from build123d import *

# Parameters (mm, degrees)
EXTRUDE_1_DEPTH   = 20
EXTRUDE_1_2_DEPTH = 55


with BuildPart() as part:
    # 草图1 → Extrude 1 (new body)
    with BuildSketch(Plane(origin=(0, 0, 0), x_dir=(1, 0, 0), z_dir=(0, 1, 0))):
        with BuildLine():
            Line((-50.205761317, 12.5), (49.794238683, 12.5))
            ThreePointArc((49.794238683, 12.5), (62.294238683, 0), (49.794238683, -12.5))
            Line((49.794238683, -12.5), (-50.205761317, -12.5))
            ThreePointArc((-50.205761317, -12.5), (-62.705761317, 0), (-50.205761317, 12.5))
        make_face()
    extrude(amount=EXTRUDE_1_DEPTH)

    # 草图2 → Extrude 1 2 (add)
    with BuildSketch(Plane(origin=(0, 20, 0), x_dir=(1, 0, 0), z_dir=(0, 1, 0))):
        with BuildLine():
            Line((49.794238683, 12.5), (-50.205761317, 12.5))
            ThreePointArc((-50.205761317, 12.5), (-62.705761317, 0), (-50.205761317, -12.5))
            Line((-50.205761317, -12.5), (49.794238683, -12.5))
            ThreePointArc((49.794238683, -12.5), (62.294238683, 0), (49.794238683, 12.5))
        make_face()
        with BuildLine():
            Line((49.794238683, 7.5), (-50.205761317, 7.5))
            ThreePointArc((-50.205761317, 7.5), (-57.705761317, 0), (-50.205761317, -7.5))
            Line((-50.205761317, -7.5), (49.794238683, -7.5))
            ThreePointArc((49.794238683, -7.5), (57.294238683, 0), (49.794238683, 7.5))
        make_face(mode=Mode.SUBTRACT)
    extrude(amount=EXTRUDE_1_2_DEPTH)


solid = part.part
Source: CAD feature listing. Evaluate the final solid. Frame: model axes, mm. A direction names the side the tool comes from. Round coordinates to 2 decimals unless told otherwise and drop trailing zeros. Order: outer loops, then holes, each group sorted by start corner. A loop starts at its lowest first (then second) coordinate and runs counter-clockwise, first axis right, second up. Notation, with made-up numbers: (38.25, -16) - (46.25, -16) arc R20 cw to (46.25, 23) - close; hole circle Ø9 at (-29, 1.5). An arc over 180 degrees is marked (long way). Use a Markdown table: item, result. Add a question column.
1. Line query: probe 1 along Z at (x, y) = (-15, 55.5); probe 2 along X at (y, z) = (59.5, -2); probe 3 along Y at (x, z) = (-7, -1.5). Output: solid intervals per line, ascending.
2. Set-up query: faces 4 (the cylindrical face through (-62.703, 36.975, -0.275)), 5 (the cylindrical face through (57.292, 47.115, 0.165)). Return all of +Z, -Z, +X, -X, +Y, -Y with unobstructed straight access to the full face (end or side cutting, diameter ignored); none if empty.
3. Section query B-B (y = 49.5). Return the cut outline in (x, z).
4. Section query A-A (x = -38). Return the cut outline in (y, z), then the cut area to 3 significant figures.
5. Section query D-D (y = 13.5). Return the cut outline in (x, z), then the cut area to 3 significant figures.
6. Mould query, pull axis X, two halves, no side actions, for faces 1 (the cylindrical face through (-57.704, 47.115, -0.165)), 2 (the flat face through (-1, 37, 12.5)), 3 (the cylindrical face through (62.29, 36.98, 0.27)). Classes: +X half, -X half, draft (parallel to the pull), parting line (faces both ways), or undercut.
7. Section query C-C (z = 0). Return the cut outline in (x, y).
8. First-contact query: pin 1 (6 mm diameter, centred on y = 34.5, z = 4, fed in from +X); pin 2 (2 mm diameter, centred on y = 29.5, z = -3, fed in from +X); pin 3 (6 mm diameter, centred on y = 32.5, z = -6, fed in from -X). Flat tips, straight axial feed; report the tip coordinate or a pass-through.
Derived:
| question | item | result |
|---|---|---|
| 1 | probe 1 | -12.5 to -7.5, 7.5 to 12.5 |
| 1 | probe 2 | -62.54 to -57.43, 57.02 to 62.13 |
| 1 | probe 3 | 0 to 20 |
| 2 | face 4 | -X, +Y, -Y |
| 2 | face 5 | +Y |
| 3 | outline | (-50.21, -12.5) - (49.79, -12.5) arc R12.5 ccw to (49.79, 12.5) - (-50.21, 12.5) arc R12.5 ccw to start; hole (-50.21, -7.5) - (49.79, -7.5) arc R7.5 ccw to (49.79, 7.5) - (-50.21, 7.5) arc R7.5 ccw to start |
| 4 | outline | (0, -12.5) - (75, -12.5) - (75, -7.5) - (20, -7.5) - (20, 7.5) - (75, 7.5) - (75, 12.5) - (0, 12.5) - close |
| 4 | area | 1,050 mm2 |
| 5 | outline | (-50.21, -12.5) - (49.79, -12.5) arc R12.5 ccw to (49.79, 12.5) - (-50.21, 12.5) arc R12.5 ccw to start |
| 5 | area | 2,990 mm2 |
| 6 | face 1 | undercut |
| 6 | face 2 | draft |
| 6 | face 3 | +X half |
| 7 | outline | (-62.71, 0) - (62.29, 0) - (62.29, 75) - (57.29, 75) - (57.29, 20) - (-57.71, 20) - (-57.71, 75) - (-62.71, 75) - close |
| 8 | pin 1 | x = 62.25 |
| 8 | pin 2 | x = 62.13 |
| 8 | pin 3 | x = -62.34 |
